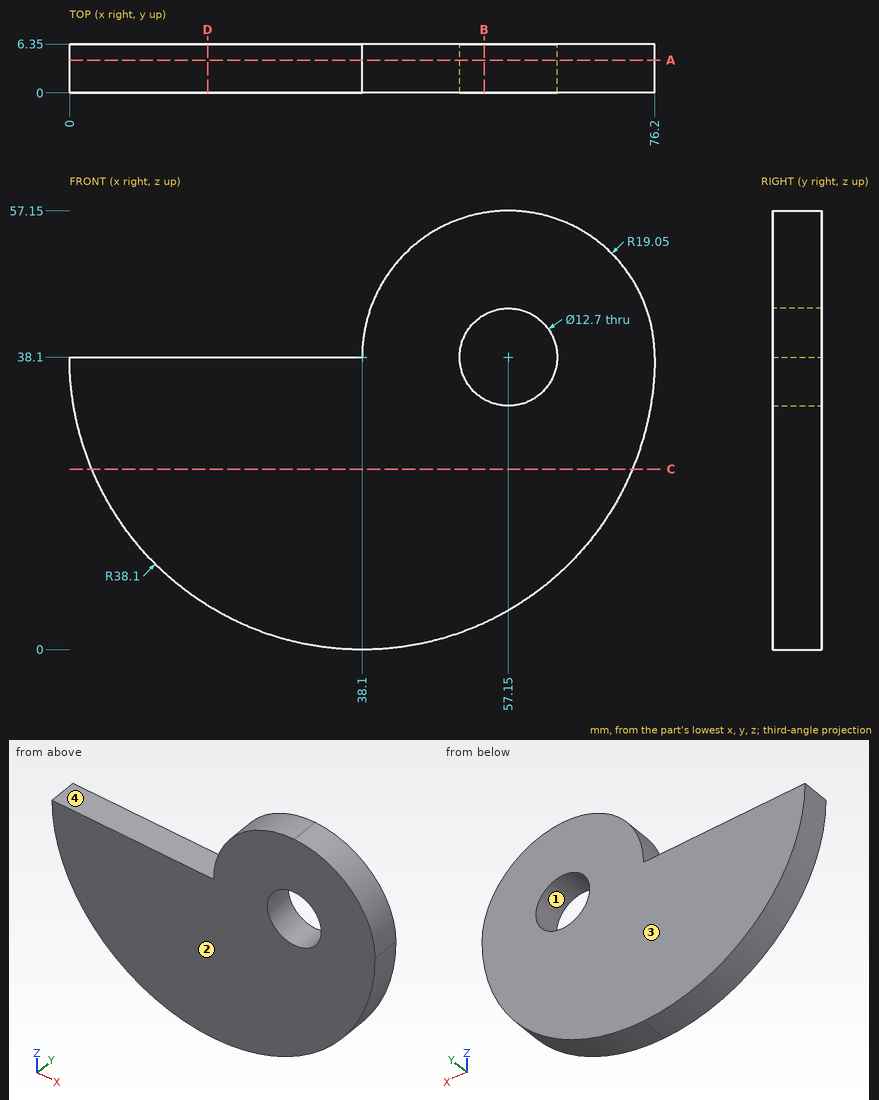
The drawing under review shows one solid part. Ordinate dimensions are in mm from its lowest x, y, z. A direction names the side the tool comes from. Coordinates: 2 decimals unless noted, no trailing zeros. Order: outer loops, then holes, each group sorted by start corner. A loop starts at its lowest first (then second) coordinate and runs counter-clockwise, first axis right, second up. Notation, with made-up numbers: M 47.25,-38 L 101.25,-38 A15 cw 101.25,-14 Z; hole C -22.5,-37 d1. An arc over 180 degrees is marked long. Use a Markdown table: item, result.
(1) Add section B-B (x = 54). Give the boundary of the cut face in (y, z), then the cut area to 3 significant figures.
Worked answers:
| item | result |
|---|---|
| outline | M 0,3.48 L 6.35,3.48 L 6.35,32.59 L 0,32.59 Z; M 0,43.61 L 6.35,43.61 L 6.35,56.89 L 0,56.89 Z |
| area | 269 mm2 |
(2) Wall thickness on probe 1 along Z at (x, y) = (56, 4.75) (3 decimals); probe 2 along X at (y, z) = (4.5, 41); probe 3 along Z at (x, y) = (53, 0.5): over which ranges is each line inside the solid? List them lowest first.
Worked answers:
| item | result |
|---|---|
| probe 1 | z = 4.467 to 31.855, 44.345 to 57.115 |
| probe 2 | x = 38.32 to 51.5, 62.8 to 75.98 |
| probe 3 | z = 3.03 to 33.29, 42.91 to 56.69 |
(3) For the marked faces 3 and 4, list the 3-axis set-ups (+Z, -Z, +X, -X, +Y, -Y) from which the entire face can be reached by the end or side of a thin tool; tool diameter is ignored.
Worked answers:
| item | result |
|---|---|
| face 3 | +Z, -Z, +X, -X, +Y |
| face 4 | +Z, -X, +Y, -Y |
(4) Add section C-C (z = 23.5). Give the boundary of the cut face in (x, y).
Worked answers:
| item | result |
|---|---|
| outline | M 2.91,0 L 73.29,0 L 73.29,6.35 L 2.91,6.35 Z |
(5) Add section A-A (y = 4.25). Give the boundary of the cut face in (x, z), then the cut area to 3 significant figures.
Worked answers:
| item | result |
|---|---|
| outline | M 0,38.1 A38.1 ccw 76.2,38.1 A19.05 ccw 38.1,38.1 Z; hole C 57.15,38.1 d12.7 |
| area | 2,720 mm2 |
(6) For P1, Ø1.9, axis at x = 18, y = 1.5, coming from the +Z side; P2, Ø7.5, axis at x = 57.15, z = 38.1, coming from the +Y side; P3, Ø1, axis at y = 3, z = 47.5, coming from the +X side, all flat-tipped, find the tip position at first contact; note any pin that passes through.
Worked answers:
| item | result |
|---|---|
| P1 | stops at z = 38.1 |
| P2 | passes through |
| P3 | stops at x = 73.99 |
(7) Add section D-D (x = 18). Give the boundary of the cut face in (y, z), then the cut area to 3 significant figures.
Worked answers:
| item | result |
|---|---|
| outline | M 0,5.73 L 6.35,5.73 L 6.35,38.1 L 0,38.1 Z |
| area | 206 mm2 |
(8) Draft analysis for pull direction X (two halves, no side actions). For the marked faces 1 and 2, state which applies: released by +X, released by -X, zero draft, split by the parting line, or undercut.
Worked answers:
| item | result |
|---|---|
| face 1 | undercut |
| face 2 | zero draft |
